from build123d import *

# Parameters (mm, degrees)
F1_DEPTH = 16
F2_DEPTH = 7
F3_DEPTH = 4
F4_R     = 2
F5_R     = 1.9999
F6_R     = 3
F7_SIZE  = 0.5


# Not quite as in the source:
# - a fillet or chamfer is up to 0.001 mm smaller than in the source, because OpenCascade refuses the exact size
# - a feature names something its author has since deleted; it is built from what else it names


with BuildPart() as f1:
    # F0 (on Front) → F1 (new body)
    with BuildSketch(Plane.XZ):
        with BuildLine():
            ThreePointArc((-5.7041860158, 8.815455853), (0, 10.5), (5.7041860158, 8.815455853))
            Line((5.7041860158, 8.815455853), (7.2831998462, 10.3944696834))
            Line((7.2831998462, 10.3944696834), (0, 17.6776695297))
            Line((0, 17.6776695297), (-7.2831998462, 10.3944696834))
            Line((-7.2831998462, 10.3944696834), (-5.7041860158, 8.815455853))
        make_face()
        with BuildLine():
            ThreePointArc((-8.815455853, 5.7041860158), (-7.4246212025, 7.4246212025), (-5.7041860158, 8.815455853))
            Line((-5.7041860158, 8.815455853), (-7.2831998462, 10.3944696834))
            Line((-7.2831998462, 10.3944696834), (-10.3944696834, 7.2831998462))
            Line((-10.3944696834, 7.2831998462), (-8.815455853, 5.7041860158))
        make_face()
        with BuildLine():
            ThreePointArc((-8.815455853, -5.7041860158), (-10.5, 0), (-8.815455853, 5.7041860158))
            Line((-8.815455853, 5.7041860158), (-10.3944696834, 7.2831998462))
            Line((-10.3944696834, 7.2831998462), (-17.6776695297, 0))
            Line((-17.6776695297, 0), (-10.3944696834, -7.2831998462))
            Line((-10.3944696834, -7.2831998462), (-8.815455853, -5.7041860158))
        make_face()
        with BuildLine():
            ThreePointArc((5.7041860158, 8.815455853), (7.4246212025, 7.4246212025), (8.815455853, 5.7041860158))
            Line((8.815455853, 5.7041860158), (10.3944696834, 7.2831998462))
            Line((10.3944696834, 7.2831998462), (7.2831998462, 10.3944696834))
            Line((7.2831998462, 10.3944696834), (5.7041860158, 8.815455853))
        make_face()
        Polygon((0, 17.6776695297), (7.2831998462, 10.3944696834), (10.111626971, 13.2228968082), (0, 23.3345237792), (-10.111626971, 13.2228968082), (-7.2831998462, 10.3944696834), align=None)
        Polygon((7.2831998462, 10.3944696834), (10.3944696834, 7.2831998462), (13.2228968082, 10.111626971), (10.111626971, 13.2228968082), align=None)
        Polygon((-10.3944696834, 7.2831998462), (-7.2831998462, 10.3944696834), (-10.111626971, 13.2228968082), (-13.2228968082, 10.111626971), align=None)
        Polygon((-17.6776695297, 0), (-10.3944696834, 7.2831998462), (-13.2228968082, 10.111626971), (-20.5060966544, 2.8284271247), (-26, 8.3223304703), (-26, 2.6654762208), (-13.2228968082, -10.111626971), (-10.3944696834, -7.2831998462), align=None)
        Polygon((-13.2228968082, 10.111626971), (-10.111626971, 13.2228968082), (-12.9400540957, 16.0513239329), (-16.0513239329, 12.9400540957), align=None)
        Polygon((17.6776695297, 0), (10.3944696834, -7.2831998462), (13.2228968082, -10.111626971), (26, 2.6654762208), (26, 8.3223304703), (20.5060966544, 2.8284271247), (13.2228968082, 10.111626971), (10.3944696834, 7.2831998462), align=None)
        with BuildLine():
            ThreePointArc((8.815455853, 5.7041860158), (10.5, 0), (8.815455853, -5.7041860158))
            Line((8.815455853, -5.7041860158), (10.3944696834, -7.2831998462))
            Line((10.3944696834, -7.2831998462), (17.6776695297, 0))
            Line((17.6776695297, 0), (10.3944696834, 7.2831998462))
            Line((10.3944696834, 7.2831998462), (8.815455853, 5.7041860158))
        make_face()
        Polygon((16.0513239329, 12.9400540957), (13.2228968082, 10.111626971), (20.5060966544, 2.8284271247), (26, 8.3223304703), (26, 12), (20, 12), (20, 30), (0, 30), (-20, 30), (-20, 12), (-26, 12), (-26, 8.3223304703), (-20.5060966544, 2.8284271247), (-13.2228968082, 10.111626971), (-16.0513239329, 12.9400540957), (-12.9400540957, 16.0513239329), (-10.111626971, 13.2228968082), (0, 23.3345237792), (10.111626971, 13.2228968082), (12.9400540957, 16.0513239329), align=None)
        Polygon((10.111626971, 13.2228968082), (13.2228968082, 10.111626971), (16.0513239329, 12.9400540957), (12.9400540957, 16.0513239329), align=None)
        Polygon((26, 2.6654762208), (13.2228968082, -10.111626971), (17.4655374953, -14.3542676581), (26, -5.8198051534), align=None)
        Polygon((-17.4655374953, -14.3542676581), (-13.2228968082, -10.111626971), (-26, 2.6654762208), (-26, -5.8198051534), align=None)
    extrude(amount=-F1_DEPTH)

    # F0 (on Front) → F2 (cut)
    with BuildSketch(Plane.XZ):
        Polygon((10.111626971, 13.2228968082), (13.2228968082, 10.111626971), (16.0513239329, 12.9400540957), (12.9400540957, 16.0513239329), align=None)
        Polygon((7.2831998462, 10.3944696834), (10.3944696834, 7.2831998462), (13.2228968082, 10.111626971), (10.111626971, 13.2228968082), align=None)
        with BuildLine():
            ThreePointArc((5.7041860158, 8.815455853), (7.4246212025, 7.4246212025), (8.815455853, 5.7041860158))
            Line((8.815455853, 5.7041860158), (10.3944696834, 7.2831998462))
            Line((10.3944696834, 7.2831998462), (7.2831998462, 10.3944696834))
            Line((7.2831998462, 10.3944696834), (5.7041860158, 8.815455853))
        make_face()
        with BuildLine():
            ThreePointArc((-8.815455853, 5.7041860158), (-7.4246212025, 7.4246212025), (-5.7041860158, 8.815455853))
            Line((-5.7041860158, 8.815455853), (-7.2831998462, 10.3944696834))
            Line((-7.2831998462, 10.3944696834), (-10.3944696834, 7.2831998462))
            Line((-10.3944696834, 7.2831998462), (-8.815455853, 5.7041860158))
        make_face()
        Polygon((-13.2228968082, 10.111626971), (-10.111626971, 13.2228968082), (-12.9400540957, 16.0513239329), (-16.0513239329, 12.9400540957), align=None)
        Polygon((-10.3944696834, 7.2831998462), (-7.2831998462, 10.3944696834), (-10.111626971, 13.2228968082), (-13.2228968082, 10.111626971), align=None)
    extrude(amount=-F2_DEPTH, mode=Mode.SUBTRACT)

    # F0 (on Front) → F3 (cut)
    with BuildSketch(Plane.XZ):
        Polygon((0, 17.6776695297), (7.2831998462, 10.3944696834), (10.111626971, 13.2228968082), (0, 23.3345237792), (-10.111626971, 13.2228968082), (-7.2831998462, 10.3944696834), align=None)
        Polygon((17.6776695297, 0), (10.3944696834, -7.2831998462), (13.2228968082, -10.111626971), (26, 2.6654762208), (26, 8.3223304703), (20.5060966544, 2.8284271247), (13.2228968082, 10.111626971), (10.3944696834, 7.2831998462), align=None)
        Polygon((-17.6776695297, 0), (-10.3944696834, 7.2831998462), (-13.2228968082, 10.111626971), (-20.5060966544, 2.8284271247), (-26, 8.3223304703), (-26, 2.6654762208), (-13.2228968082, -10.111626971), (-10.3944696834, -7.2831998462), align=None)
    extrude(amount=-F3_DEPTH, mode=Mode.SUBTRACT)

    # F4
    f4_edges = [f1.edges().sort_by_distance(p)[0] for p in [
        (-16.051324, 3.5, 12.940054),
        (-12.940054, 3.5, 16.051324),
        (12.940054, 3.5, 16.051324),
        (16.051324, 3.5, 12.940054),
        (0, 2, 23.334524),
    ]]
    fillet(f4_edges, radius=F4_R)

    # F5 (radius 2 in the source; OpenCascade refuses exactly that, so slightly less here)
    f5_edges = [f1.edges().sort_by_distance(p)[0] for p in [
        (19.611448, 4, -3.723075),
        (14.03607, 4, -3.6416),
        (14.03607, 4, 3.6416),
        (16.864497, 4, 6.470027),
        (5.76292, 4, 17.571604),
        (-16.864497, 4, 6.470027),
        (-23.253048, 4, 5.575379),
        (-14.03607, 4, -3.6416),
        (-3.6416, 4, 14.03607),
        (-14.03607, 4, 3.6416),
        (-19.611448, 4, -3.723075),
        (23.253048, 4, 5.575379),
        (0, 4, 22.506097),
        (-5.76292, 4, 17.571604),
        (3.6416, 4, 14.03607),
    ]]
    fillet(f5_edges, radius=F5_R)

    # F6
    f6_edges = [f1.edges().sort_by_distance(p)[0] for p in [
        (17.465537, 8, -14.354268),
        (26, 8, -5.819805),
        (-26, 8, -5.819805),
        (-17.465537, 8, -14.354268),
    ]]
    fillet(f6_edges, radius=F6_R)

    # F7
    f7_edges = [f1.edges().sort_by_distance(p)[0] for p in [
        (20, 8, 30),
        (26, 8, 12),
        (-20, 8, 30),
        (-26, 8, 12),
    ]]
    chamfer(f7_edges, length=F7_SIZE)


solid = f1.part
Model file for the job. Use its own axes, mm. A direction names the side the tool comes from. Round coordinates to 2 decimals unless told otherwise and drop trailing zeros. Loops run counter-clockwise (first coordinate to the right, second up) from the corner with the lowest first, then second, coordinate; pieces in that order, holes last. Notation, with made-up numbers: (40.25, 32) -> (83.25, 32) arc R15 ccw to (83.25, 47) -> close; hole circle Ø9 at (56, 49.25). An arc over 180 degrees is marked (long way). Answer as CSV lines item,"result". Start each with the question number.
1) Slice it at B-B (y = 13). List the corners of the cut face in (x, z), plus the area to 3 significant figures.
2) Mould opens along X. For faces 5 (the face through (22.32, 7.89, -9.5)), 6 (the face through (-21, 0, -7)), 7 (the face through (-14.09, 0.99, 3.59)) say: +X half, -X half, draft (parallel to the pull), parting line (faces both ways), or undercut.
3) Probe line 1 along X through (y, z) = (6.25, 13); line 2 along Z through (x, y) = (9.5, 8); line 3 along X through (y, z) = (6.5, 4). List the from-to ranges inside material, lowest first.
4) Tool access for faces 1 (the face through (23.29, 0.99, 5.61)), 2 (the face through (20, 8, 21)), 3 (the face through (-12.126, 7.888, -9.014)), 4 (the face through (-17.23, 3.4, 5.3)): list every direction of +Z, -Z, +X, -X, +Y, -Y with a clear straight run to the whole face (end or side of a thin tool).
5) Pin check, flat tips, straight feed: P1, Ø4.5, axis at x = 20, z = -1, coming from the -Y side; P2, Ø1.6, axis at x = -23.5, y = 6, coming from the +Z side; P3, Ø1.5, axis at x = -6.5, y = 3, coming from the -Z side; P4, Ø5, axis at y = 6, z = 17, coming from the -X side. Stop position of each tip, or through.
Filled in:
1,outline,"(-26, -4.58) arc R3 ccw to (-25.12, -6.7) -> (-19.59, -12.23) arc R3 ccw to (-15.34, -12.23) -> (-8.82, -5.7) arc R10.5 cw (long way) to (8.82, -5.7) -> (15.34, -12.23) arc R3 ccw to (19.59, -12.23) -> (25.12, -6.7) arc R3 ccw to (26, -4.58) -> (26, 11.5) -> (25.5, 12) -> (20, 12) -> (20, 29.5) -> (19.5, 30) -> (-19.5, 30) -> (-20, 29.5) -> (-20, 12) -> (-25.5, 12) -> (-26, 11.5) -> close"
1,area,"1,500 mm2"
2,face 5,"+X half"
2,face 6,"draft"
2,face 7,"undercut"
3,line 1,"x = -20 to -15.22, -9.89 to 9.89, 15.22 to 20"
3,line 2,"z = -6.39 to -4.47, 4.47 to 30"
3,line 3,"x = -26 to -9.71, 9.71 to 26"
4,face 1,"+X, -Y"
4,face 2,"+Z, +X, +Y, -Y"
4,face 3,"-Z, +Y, -Y"
4,face 4,"-Y"
5,P1,"stops at y = 0"
5,P2,"stops at z = 12"
5,P3,"stops at z = 8.86"
5,P4,"stops at x = -20"
